The listing builds one solid part. Answer for the finished solid, in the listing's coordinates (mm). Face numbers are marked on the shaded views. A direction names the side the tool comes from. Coordinates: 2 decimals unless noted, no trailing zeros. Loops run counter-clockwise (first coordinate to the right, second up) from the corner with the lowest first, then second, coordinate; pieces in that order, holes last. Notation, with made-up numbers: (-33, 58) - (19, 58) arc R26 cw to (19, 83) - close; hole circle Ø11 at (86.5, 75). An arc over 180 degrees is marked (long way). Put each result on its own line as item: value.
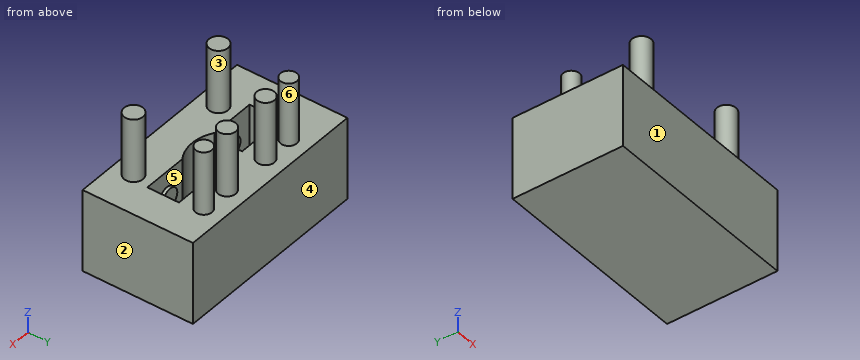
```python
from build123d import *

# Parameters (mm, degrees)
SKETCH1_R      = 24
EXTRUDE1_DEPTH = 5
SKETCH2_R      = 24
EXTRUDE2_DEPTH = 8
SKETCH9_R      = 24
SKETCH9_W      = 31.75
SKETCH9_H      = 17.4625
EXTRUDE4_DEPTH = 13
SKETCH10_R     = 1.3
SKETCH10_R_2   = 1.5
SKETCH10_R_3   = 1.4
EXTRUDE5_DEPTH = 10
SKETCH11_R     = 1.5
EXTRUDE6_DEPTH = 0.5


with BuildPart() as part:
    # Sketch1 → Extrude1 (new body)
    with BuildSketch(Plane.XY):
        Circle(SKETCH1_R)
    extrude(amount=EXTRUDE1_DEPTH)

    # Sketch2 → Extrude2 (add)
    with BuildSketch(Plane.XY.offset(5)):
        Circle(SKETCH2_R)
        with BuildLine():
            Line((-2.5, 0), (-10.5, 0))
            Line((-10.5, 0), (-10.5, -5))
            Line((-10.5, -5), (-3.31662479, -5))
            ThreePointArc((-3.31662479, -5), (0, -6), (3.31662479, -5))
            Line((3.31662479, -5), (10.5, -5))
            Line((10.5, -5), (10.5, 0))
            Line((10.5, 0), (2.5, 0))
            ThreePointArc((2.5, 0), (0, -2.5), (-2.5, 0))
        make_face(mode=Mode.SUBTRACT)
    extrude(amount=EXTRUDE2_DEPTH)

    # Sketch9 → Extrude4 (cut)
    with BuildSketch(Plane.XY.offset(13)):
        Circle(SKETCH9_R)
        with Locations((0, -2.38125)):
            Rectangle(SKETCH9_W, SKETCH9_H, mode=Mode.SUBTRACT)
    extrude(amount=-EXTRUDE4_DEPTH, mode=Mode.SUBTRACT)

    # Sketch10 → Extrude5 (add)
    with BuildSketch(Plane.XY.offset(13)):
        with Locations((9.525, 3.175)):
            Circle(SKETCH10_R)
        with Locations((-7.9375, 3.175)):
            Circle(SKETCH10_R)
        with Locations((-7.9375, -7.9375)):
            Circle(SKETCH10_R_2)
        with Locations((9.525, -7.9375)):
            Circle(SKETCH10_R_2)
        with Locations((-3.175, 3.175)):
            Circle(SKETCH10_R_3)
        with Locations((4.7625, 3.175)):
            Circle(SKETCH10_R_3)
    extrude(amount=EXTRUDE5_DEPTH)

    # Sketch11 → Extrude6 (add)
    with BuildSketch(Plane(origin=(0, -5, 0), x_dir=(1, 0, 0), z_dir=(0, 1, 0))):
        with Locations((-6.5, -9)):
            Circle(SKETCH11_R)
        with Locations((6.5, -9)):
            Circle(SKETCH11_R)
    extrude(amount=EXTRUDE6_DEPTH)


solid = part.part
```
1) Each of these flat-tipped pins is pushed along its axis until it touches: pin 1 (1 mm diameter, centred on x = 7.5, y = -8.5, fed in from +Z); pin 2 (5 mm diameter, centred on y = -3.5, z = 14.5, fed in from +X) (3 decimals); pin 3 (4 mm diameter, centred on x = 2, z = 20, fed in from -Y). Where does it stop, or does it pass through?
Found:
pin 1: stops at z = 13
pin 2: stops at x = 15.875
pin 3: stops at y = 2
2) For a pull along Y with two mould halves and no side action, classify the marked faces 1, 2 and 3 as pulls with the +Y half, pulls with the -Y half, needs draft (parallel to the pull), parting line crosses it, or undercut.
Found:
face 1: pulls with the -Y half
face 2: needs draft
face 3: undercut
3) The part is cut by section C-C (x = 0). Give the vertices of the cut face in (y, z), and give its area (3 significant figures).
Found:
outline: (-11.11, 0) - (6.35, 0) - (6.35, 13) - (-2.5, 13) - (-2.5, 5) - (-6, 5) - (-6, 13) - (-11.11, 13) - close
area: 199 mm^2
4) Straight lines are drawn through the part: L1, parallel to Y at x = 5, z = 8; L2, parallel to Z at x = 14.5, y = -0.75; L3, parallel to Z at x = -1, y = -2.5. For each, find the intervals that lie inside material, in ascending order. Write a range as [from, to].
Found:
L1: y = [-11.11, -5], [0, 6.35]
L2: z = [0, 13]
L3: z = [0, 5]
5) For the marked faces 4, 5 and 6, determine the directions among +Z, -Z, +X, -X, +Y, -Y from which every point of the face is accessible in a straight line to the end or side of a thin tool.
Found:
face 4: +Z, -Z, +X, -X, +Y
face 5: none
face 6: +Z
6) The part is cut by section B-B (y = -4). Give the vertices of the cut face in (x, z) (3 decimals), and give its area (3 significant figures).
Found:
outline: (-15.875, 0) - (15.875, 0) - (15.875, 13) - (10.5, 13) - (10.5, 5) - (-10.5, 5) - (-10.5, 13) - (-15.875, 13) - close
area: 245 mm^2
